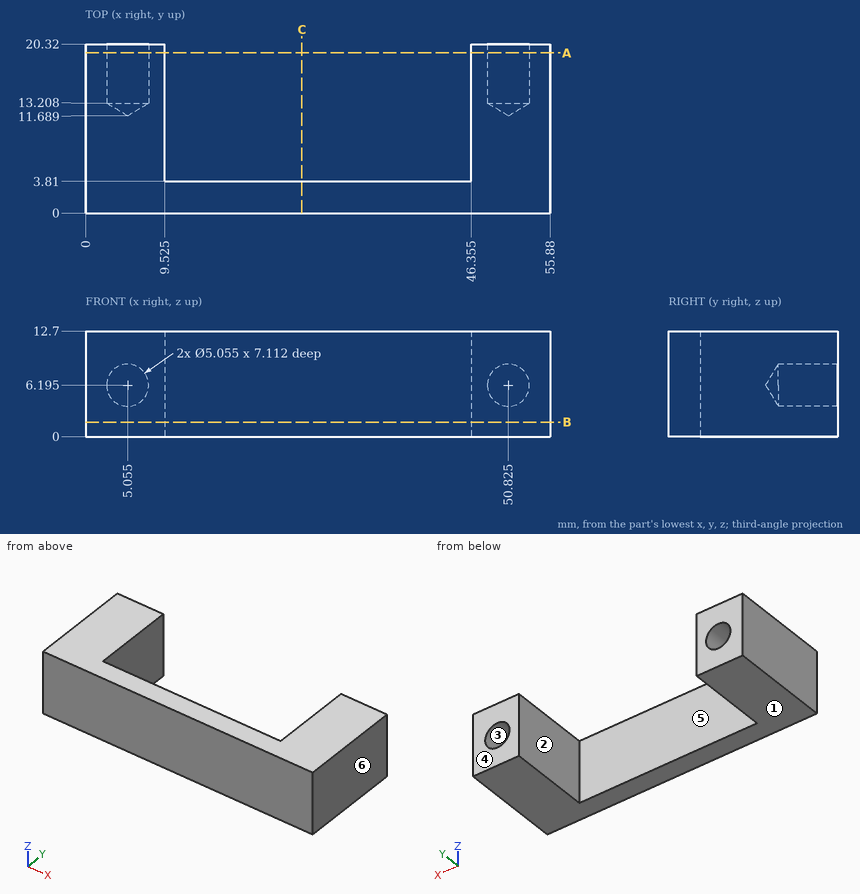
Verification items for this drawing (mm, ordinates from the low corner). A direction names the side the tool comes from. Round coordinates to 2 decimals unless told otherwise and drop trailing zeros. Loops run counter-clockwise (first coordinate to the right, second up) from the corner with the lowest first, then second, coordinate; pieces in that order, holes last. Notation, with made-up numbers: (38, -4.75) -> (45, -4.75) arc R35 cw to (45, 28.25) -> close; hole circle Ø6 at (36.25, -19.75). An arc over 180 degrees is marked (long way). Write item = value, one per line. Start each with the question number.
1) Thickness scan on probe 1 along X at (y, z) = (5, 11.25) (1 decimal); probe 2 along X at (y, z) = (18.5, 7.5) (1 decimal); probe 3 along X at (y, z) = (19, 6) (1 decimal). Record the ranges inside material, lowest first.
2) Sectioned sample at C-C, the plane x = 26. Record the cut outline in (y, z), plus the area to 3 significant figures.
3) Sectioned sample at A-A, the plane y = 19.25. Record the cut outline in (x, z) (1 decimal), plus the area to 3 significant figures.
4) Sectioned sample at B-B, the plane z = 1.75. Record the cut outline in (x, y) (1 decimal).
5) Release check for a two-part mould opening along X. For the marked faces 4, 5 and 6 record: released by +X, released by -X, zero draft, split by the parting line, or undercut.
6) Gauge pin test, flat end, axial feed: pin 1 Ø4 at (x, z) = (5.05, 6.19) entering from +Y (1 decimal). Record the tip position at first contact, or that the pin passes through.
7) Set-up check for the marked faces 1, 2 and 3: record each of +Z, -Z, +X, -X, +Y, -Y from which the full face is reachable in a straight line by a thin tool's end or side.
Results are:
q1.probe_1 = 0 to 9.5, 46.4 to 55.9
q1.probe_2 = 0 to 2.9, 7.2 to 9.5, 46.4 to 48.7, 53 to 55.9
q1.probe_3 = 0 to 2.5, 7.6 to 9.5, 46.4 to 48.3, 53.3 to 55.9
q2.outline = (0, 0) -> (3.81, 0) -> (3.81, 12.7) -> (0, 12.7) -> close
q2.area = 48.4 mm^2
q3.outline = (0, 0) -> (9.5, 0) -> (9.5, 12.7) -> (0, 12.7) -> close; (46.4, 0) -> (55.9, 0) -> (55.9, 12.7) -> (46.4, 12.7) -> close; hole circle Ø5.1 at (5.1, 6.2); hole circle Ø5.1 at (50.8, 6.2)
q3.area = 202 mm^2
q4.outline = (0, 0) -> (55.9, 0) -> (55.9, 20.3) -> (46.4, 20.3) -> (46.4, 3.8) -> (9.5, 3.8) -> (9.5, 20.3) -> (0, 20.3) -> close
q5.face_4 = zero draft
q5.face_5 = undercut
q5.face_6 = released by +X
q6.pin_1 = 12.9
q7.face_1 = -Z, +X, -X, +Y, -Y
q7.face_2 = +Z, -Z, +Y
q7.face_3 = +Y
